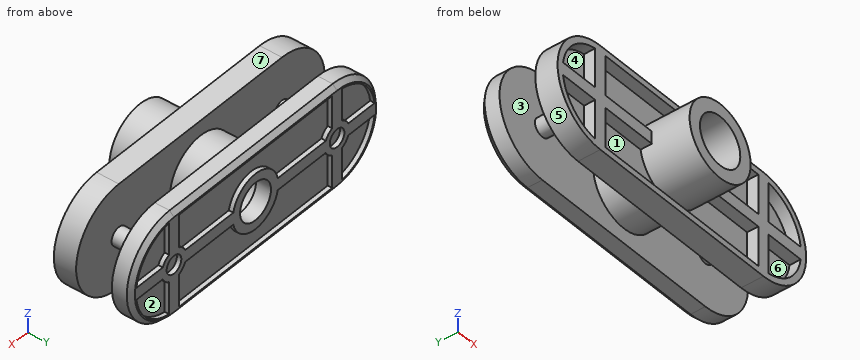
```python
from build123d import *

# Parameters (mm, degrees)
SALIENTE_EXTRUIR1_DEPTH = 1.3
CROQUIS2_R              = 0.6
CORTAR_EXTRUIR1_DEPTH   = 0.3
CHAFL_N1_SIZE           = 0.3
SALIENTE_EXTRUIR2_REACH = 13.047
CROQUIS3_R              = 0.6
CROQUIS3_R_2            = 2.5
SALIENTE_EXTRUIR3_START = -1.2
CROQUIS4_R              = 0.6
CROQUIS4_R_2            = 2.5
SALIENTE_EXTRUIR3_DEPTH = 1.2
SALIENTE_EXTRUIR4_START = 1.5
SALIENTE_EXTRUIR4_DEPTH = 1.5
CROQUIS6_W              = 12.51
CROQUIS6_H              = 2.66
CORTAR_EXTRUIR3_DEPTH   = 0.75
SALIENTE_EXTRUIR5_START = 3.32
CROQUIS8_R              = 2.5
SALIENTE_EXTRUIR5_DEPTH = 3.32
CROQUIS9_R              = 1.65
CORTAR_EXTRUIR4_DEPTH   = 6.77
CROQUIS10_R             = 1.265
CORTAR_EXTRUIR6_DEPTH   = 6.77
CROQUIS12_R             = 1.865
CROQUIS12_R_2           = 1.265
SALIENTE_EXTRUIR6_DEPTH = 0.3


with BuildPart() as part:
    # Croquis1 → Saliente-Extruir1 (new body)
    with BuildSketch(Plane(origin=(0, 0, 0), x_dir=(1, 0, 0), z_dir=(0, 1, 0))):
        with BuildLine():
            Line((-6.675, 3.5), (6.675, 3.5))
            ThreePointArc((6.675, 3.5), (10.175, 0), (6.675, -3.5))
            Line((6.675, -3.5), (-6.675, -3.5))
            ThreePointArc((-6.675, -3.5), (-10.175, 0), (-6.675, 3.5))
        make_face()
    extrude(amount=SALIENTE_EXTRUIR1_DEPTH)

    # Croquis2 → Cortar-Extruir1 (cut)
    with BuildSketch(Plane(origin=(0, 1.3, 0), x_dir=(1, 0, 0), z_dir=(0, 1, 0))):
        with Locations(Location((-6.675, 0, 0), (0, 0, 270))):
            Circle(CROQUIS2_R)
        with Locations(Location((6.675, 0, 0), (0, 0, 90))):
            Circle(CROQUIS2_R)
        with BuildLine():
            Line((-7.075, 3.07408523), (-7.075, 0.916515139))
            ThreePointArc((-7.075, 0.916515139), (-7.382106781, 0.707106781), (-7.591515139, 0.4))
            Line((-7.591515139, 0.4), (-9.74908523, 0.4))
            ThreePointArc((-9.74908523, 0.4), (-8.867031022, 2.192031022), (-7.075, 3.07408523))
        make_face()
        with BuildLine():
            Line((-6.275, 3.1), (-6.275, 0.916515139))
            ThreePointArc((-6.275, 0.916515139), (-5.967893219, 0.707106781), (-5.758484861, 0.4))
            Line((-5.758484861, 0.4), (5.758484861, 0.4))
            ThreePointArc((5.758484861, 0.4), (5.967893219, 0.707106781), (6.275, 0.916515139))
            Line((6.275, 0.916515139), (6.275, 3.1))
            Line((6.275, 3.1), (-6.275, 3.1))
        make_face()
        with BuildLine():
            Line((-6.275, -0.916515139), (-6.275, -3.1))
            Line((-6.275, -3.1), (6.275, -3.1))
            Line((6.275, -3.1), (6.275, -0.916515139))
            ThreePointArc((6.275, -0.916515139), (5.967893219, -0.707106781), (5.758484861, -0.4))
            Line((5.758484861, -0.4), (-5.758484861, -0.4))
            ThreePointArc((-5.758484861, -0.4), (-5.967893219, -0.707106781), (-6.275, -0.916515139))
        make_face()
        with BuildLine():
            Line((-7.591515139, -0.4), (-9.74908523, -0.4))
            ThreePointArc((-9.74908523, -0.4), (-8.867031022, -2.192031022), (-7.075, -3.07408523))
            Line((-7.075, -3.07408523), (-7.075, -0.916515139))
            ThreePointArc((-7.075, -0.916515139), (-7.382106781, -0.707106781), (-7.591515139, -0.4))
        make_face()
        with BuildLine():
            Line((7.075, -0.916515139), (7.075, -3.07408523))
            ThreePointArc((7.075, -3.07408523), (8.867031022, -2.192031022), (9.74908523, -0.4))
            Line((9.74908523, -0.4), (7.591515139, -0.4))
            ThreePointArc((7.591515139, -0.4), (7.382106781, -0.707106781), (7.075, -0.916515139))
        make_face()
        with BuildLine():
            Line((7.591515139, 0.4), (9.74908523, 0.4))
            ThreePointArc((9.74908523, 0.4), (8.867031022, 2.192031022), (7.075, 3.07408523))
            Line((7.075, 3.07408523), (7.075, 0.916515139))
            ThreePointArc((7.075, 0.916515139), (7.382106781, 0.707106781), (7.591515139, 0.4))
        make_face()
    extrude(amount=-CORTAR_EXTRUIR1_DEPTH, mode=Mode.SUBTRACT)

    # Chaflán1
    chafl_n1_edges = [part.edges().sort_by_distance(p)[0] for p in [
        (10.175, 1.3, 0),
        (0, 1.3, -3.5),
        (-10.175, 1.3, 0),
        (0, 1.3, 3.5),
    ]]
    chamfer(chafl_n1_edges, length=CHAFL_N1_SIZE)

    # Croquis3 → Saliente-Extruir2 (add, up to next)
    with BuildSketch(Plane(origin=(0, -1.2, 0), x_dir=(1, 0, 0), z_dir=(0, 1, 0)), mode=Mode.PRIVATE) as saliente_extruir2_sk1:
        with Locations(Location((6.675, 0, 0), (0, 0, 90))):
            Circle(CROQUIS3_R)
    saliente_extruir2_tool1 = extrude(saliente_extruir2_sk1.sketch, amount=SALIENTE_EXTRUIR2_REACH, mode=Mode.PRIVATE) - part.part
    # Croquis3 → Saliente-Extruir2 (add, up to next)
    with BuildSketch(Plane(origin=(0, -1.2, 0), x_dir=(1, 0, 0), z_dir=(0, 1, 0)), mode=Mode.PRIVATE) as saliente_extruir2_sk2:
        with Locations(Location((-6.675, 0, 0), (0, 0, 270))):
            Circle(CROQUIS3_R)
    saliente_extruir2_tool2 = extrude(saliente_extruir2_sk2.sketch, amount=SALIENTE_EXTRUIR2_REACH, mode=Mode.PRIVATE) - part.part
    # Croquis3 → Saliente-Extruir2 (add, up to next)
    with BuildSketch(Plane(origin=(0, -1.2, 0), x_dir=(1, 0, 0), z_dir=(0, 1, 0)), mode=Mode.PRIVATE) as saliente_extruir2_sk3:
        with Locations(Location((0, 0, 0), (0, 0, 270))):
            Circle(CROQUIS3_R_2)
    saliente_extruir2_tool3 = extrude(saliente_extruir2_sk3.sketch, amount=SALIENTE_EXTRUIR2_REACH, mode=Mode.PRIVATE) - part.part
    add(saliente_extruir2_tool1.solids().sort_by_distance((6.675, -1.2, 0))[0])
    add(saliente_extruir2_tool2.solids().sort_by_distance((-6.675, -1.2, 0))[0])
    add(saliente_extruir2_tool3.solids().sort_by_distance((0, -1.2, 0))[0])

    # Croquis4 → Saliente-Extruir3 (add)
    with BuildSketch(Plane(origin=(0, -1.2, 0), x_dir=(1, 0, 0), z_dir=(0, 1, 0)).offset(SALIENTE_EXTRUIR3_START)):
        with Locations(Location((6.675, 0, 0), (0, 0, 90))):
            Circle(CROQUIS4_R)
        with Locations(Location((-6.675, 0, 0), (0, 0, 270))):
            Circle(CROQUIS4_R)
        with Locations(Location((0, 0, 0), (0, 0, 270))):
            Circle(CROQUIS4_R_2)
    extrude(amount=SALIENTE_EXTRUIR3_DEPTH)

    # Croquis5 → Saliente-Extruir4 (add)
    with BuildSketch(Plane.XZ.offset(2.4).offset(SALIENTE_EXTRUIR4_START)):
        with BuildLine():
            Line((6.675, -3.5), (-6.675, -3.5))
            ThreePointArc((-6.675, -3.5), (-10.175, 0), (-6.675, 3.5))
            Line((-6.675, 3.5), (6.675, 3.5))
            ThreePointArc((6.675, 3.5), (10.175, 0), (6.675, -3.5))
        make_face()
    extrude(amount=-SALIENTE_EXTRUIR4_DEPTH)

    # Croquis6 → Cortar-Extruir3 (cut)
    with BuildSketch(Plane.XZ.offset(3.9)):
        with Locations((0, 1.75)):
            Rectangle(CROQUIS6_W, CROQUIS6_H)
        with BuildLine():
            Line((-9.72622926, -0.42), (-7.095, -0.42))
            Line((-7.095, -0.42), (-7.095, -3.05122926))
            ThreePointArc((-7.095, -3.05122926), (-8.852888886, -2.177888886), (-9.72622926, -0.42))
        make_face()
        with Locations((0, -1.75)):
            Rectangle(CROQUIS6_W, CROQUIS6_H)
        with BuildLine():
            Line((7.095, -3.05122926), (7.095, -0.42))
            Line((7.095, -0.42), (9.72622926, -0.42))
            ThreePointArc((9.72622926, -0.42), (8.852888886, -2.177888886), (7.095, -3.05122926))
        make_face()
        with BuildLine():
            Line((-9.72622926, 0.42), (-7.095, 0.42))
            Line((-7.095, 0.42), (-7.095, 3.05122926))
            ThreePointArc((-7.095, 3.05122926), (-8.852888886, 2.177888886), (-9.72622926, 0.42))
        make_face()
        with BuildLine():
            Line((7.095, 0.42), (9.72622926, 0.42))
            ThreePointArc((9.72622926, 0.42), (8.852888886, 2.177888886), (7.095, 3.05122926))
            Line((7.095, 3.05122926), (7.095, 0.42))
        make_face()
    extrude(amount=-CORTAR_EXTRUIR3_DEPTH, mode=Mode.SUBTRACT)

    # Croquis8 → Saliente-Extruir5 (add)
    with BuildSketch(Plane.XZ.offset(3.15).offset(SALIENTE_EXTRUIR5_START)):
        with Locations(Location((0, 0, 0), (0, 0, 90))):
            Circle(CROQUIS8_R)
    extrude(amount=-SALIENTE_EXTRUIR5_DEPTH)

    # Croquis9 → Cortar-Extruir4 (cut)
    with BuildSketch(Plane.XZ.offset(6.47)):
        with Locations(Location((0, 0, 0), (0, 0, 270))):
            Circle(CROQUIS9_R)
    extrude(amount=-CORTAR_EXTRUIR4_DEPTH, mode=Mode.SUBTRACT)

    # Croquis10 → Cortar-Extruir6 (cut)
    with BuildSketch(Plane.XZ.offset(-0.3)):
        with Locations(Location((0, 0, 0), (0, 0, 270))):
            Circle(CROQUIS10_R)
    extrude(amount=-CORTAR_EXTRUIR6_DEPTH, mode=Mode.SUBTRACT)

    # Croquis12 → Saliente-Extruir6 (add)
    with BuildSketch(Plane(origin=(0, 1, 0), x_dir=(1, 0, 0), z_dir=(0, 1, 0))):
        Circle(CROQUIS12_R)
        with Locations(Location((0, 0, 0), (0, 0, 90))):
            Circle(CROQUIS12_R_2, mode=Mode.SUBTRACT)
    extrude(amount=SALIENTE_EXTRUIR6_DEPTH)


solid = part.part
```
The model under review builds one solid part; all positions refer to its coordinate system, in mm. Face numbers are marked on the shaded views. A direction names the side the tool comes from. Round coordinates to 2 decimals unless told otherwise and drop trailing zeros. Loops run counter-clockwise (first coordinate to the right, second up) from the corner with the lowest first, then second, coordinate; pieces in that order, holes last.
1) Consider section B-B on z = 0. Give the number of separate pieces and of enclosed holes in the cut face, then the cut area to 3 significant figures.
Values follow:
separate pieces: 2
enclosed holes: 2
area: 61.9 mm2
2) Consider section C-C on y = -2. State the section outline as (x, z) points (3 decimals).
Values follow:
outline: circle Ø1.2 at (-6.675, 0); circle Ø5 at (0, 0); circle Ø1.2 at (6.675, 0); hole circle Ø3.3 at (0, 0)
3) Consider section D-D on y = -5.5. State the section outline as (x, z) points, then the cut area to 3 significant figures.
Values follow:
outline: circle Ø5 at (0, 0); hole circle Ø3.3 at (0, 0)
area: 11.1 mm2
4) Tool access review of the marked faces 1, 2 and 3: name each direction out of +Z, -Z, +X, -X, +Y, -Y from which nothing blocks a thin tool from reaching the whole face with its end or side.
Values follow:
face 1: -Y
face 2: +Y
face 3: none
5) Wall thickness on line 1 along Z through (x, y) = (3, -3.75); line 2 along Y through (x, z) = (-7, -2.75); line 3 along Y through (x, z) = (-4.75, -2.75): over which ranges is each line inside the solid? List them lowest first.
Values follow:
line 1: z = -3.5 to -3.08, -0.42 to 0.42, 3.08 to 3.5
line 2: y = -3.9 to -2.4, 0 to 1.3
line 3: y = -3.15 to -2.4, 0 to 1
6) Clearance check with flat-ended pins moving along their axes: P1, Ø4, axis at y = -5, z = -2, coming from the -X side; P2, Ø0.6, axis at y = -3.5, z = 1.5, coming from the +X side; P3, Ø0.8, axis at x = 2.5, z = 1.5, coming from the +Y side. State where each tip first meets the part, or that it passes through.
Values follow:
P1: stops at x = -10.16
P2: stops at x = 9.96
P3: stops at y = 1
7) Consider section A-A on x = -4.75. State the section outline as (y, z) points.
Values follow:
outline: (-3.9, -3.5) - (-2.4, -3.5) - (-2.4, 3.5) - (-3.9, 3.5) - (-3.9, 3.08) - (-3.15, 3.08) - (-3.15, 0.42) - (-3.9, 0.42) - (-3.9, -0.42) - (-3.15, -0.42) - (-3.15, -3.08) - (-3.9, -3.08) - close; (0, -3.5) - (1, -3.5) - (1.3, -3.2) - (1.3, -3.1) - (1, -3.1) - (1, -0.4) - (1.3, -0.4) - (1.3, 0.4) - (1, 0.4) - (1, 3.1) - (1.3, 3.1) - (1.3, 3.2) - (1, 3.5) - (0, 3.5) - close
8) The part is to be moulded in two halves that separate along X. For the marked faces 4, 5, 6 and 7, say which applies: pulls with the +X half, pulls with the -X half, needs draft (parallel to the pull), parting line crosses it, or undercut.
Values follow:
face 4: undercut
face 5: pulls with the -X half
face 6: undercut
face 7: needs draft
